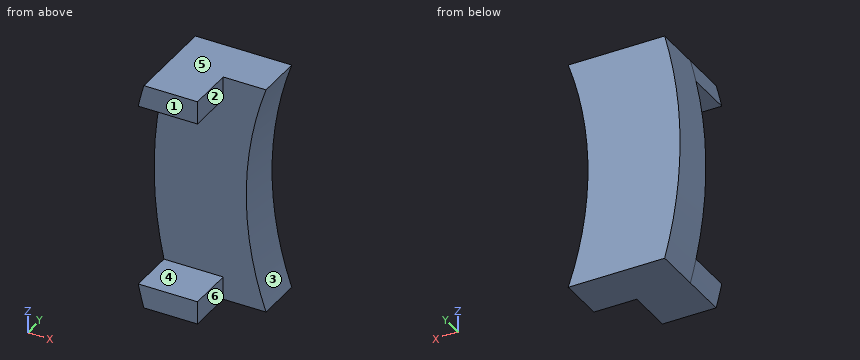
```python
from build123d import *

# Parameters (mm, degrees)
BOSS_EXTRUDE1_DEPTH = 2
BOSS_EXTRUDE2_DEPTH = 2


with BuildPart() as part:
    # Sketch1 → Boss-Extrude1 (new body)
    with BuildSketch(Plane(origin=(0, 0, 0), x_dir=(1, 0, 0), z_dir=(0, 1, 0))):
        with BuildLine():
            Line((-18.33030278, 5), (-14.142135624, 5))
            ThreePointArc((-14.142135624, 5), (-15, 0), (-14.142135624, -5))
            Line((-14.142135624, -5), (-18.33030278, -5))
            ThreePointArc((-18.33030278, -5), (-19, 0), (-18.33030278, 5))
        make_face()
    extrude(amount=BOSS_EXTRUDE1_DEPTH)

    # Sketch2 → Boss-Extrude2 (add)
    with BuildSketch(Plane.XZ):
        with BuildLine():
            Line((-16, -5), (-18.33030278, -5))
            ThreePointArc((-18.33030278, -5), (-18.459012203, -4.501651751), (-18.574175621, -4))
            Line((-18.574175621, -4), (-16, -4))
            Line((-16, -4), (-16, -5))
        make_face()
        with BuildLine():
            Line((-18.33030278, 5), (-16, 5))
            Line((-16, 5), (-16, 4))
            Line((-16, 4), (-18.574175621, 4))
            ThreePointArc((-18.574175621, 4), (-18.459012203, 4.501651751), (-18.33030278, 5))
        make_face()
    extrude(amount=BOSS_EXTRUDE2_DEPTH)


solid = part.part
```
CAD build for the part. Positions are in the model's coordinates, mm. Face numbers are marked on the shaded views. A direction names the side the tool comes from. Round coordinates to 2 decimals unless told otherwise and drop trailing zeros. Write each loop counter-clockwise with the first axis right and the second up, starting at its lowest first coordinate (ties: lowest second). Pieces come first, ordered by that corner, then holes. Notation, with made-up numbers: (-38, 82.5) -> (-22, 82.5) arc R16 cw to (-22, 95.5) -> close; hole circle Ø8 at (85, -18). An arc over 180 degrees is marked (long way). Answer in a Markdown table with one row per item. Add a question column.
Item 1: Mould opens along Z. For the marked faces 3, 4, 5 and 6 say: pulls with the +Z half, pulls with the -Z half, needs draft (parallel to the pull), parting line crosses it, or undercut.
Item 2: Saw through at B-B, the plane x = -17.4. Write the cut outline in (y, z).
Item 3: Drop flat-ended pins along their axis: pin 1 Ø1 at (y, z) = (0.5, -4) entering from +X; pin 2 Ø0.5 at (y, z) = (-1.5, -4.5) entering from +X; pin 3 Ø1 at (x, z) = (-16, -0.5) entering from -Y. Give the stop position or say it passes through.
Item 4: Drill centre lines: line 1 (Z direction, x = -17.2, y = -1.75); line 2 (Y direction, x = -18.3, z = 1); line 3 (X direction, y = 0.3, z = -0.75). Where is each one in solid material? Low to high. Write a range as from..to.
Item 5: Saw through at C-C, the plane x = -14.45. Write the cut outline in (y, z), then the cut area to 3 significant figures.
Item 6: Which spindle directions (+Z, -Z, +X, -X, +Y, -Y) get a long thin tool onto all of the face, cutting with end or side? Do the marked faces 1 and 2. Say none if no direction does.
Item 7: Saw through at A-A, the plane y = -1.05. Write the cut outline in (x, z), then the cut area to 3 significant figures.
Item 8: Saw through at D-D, the plane z = 0. Write the cut outline in (x, y), then the cut area to 3 significant figures.
Findings below:
| question | item | result |
|---|---|---|
| 1 | face 3 | undercut |
| 1 | face 4 | undercut |
| 1 | face 5 | pulls with the +Z half |
| 1 | face 6 | needs draft |
| 2 | outline | (-2, -5) -> (2, -5) -> (2, 5) -> (-2, 5) -> (-2, 4) -> (0, 4) -> (0, -4) -> (-2, -4) -> close |
| 3 | pin 1 | stops at x = -14.31 |
| 3 | pin 2 | stops at x = -16 |
| 3 | pin 3 | stops at y = 0 |
| 4 | line 1 | z = -5..-4, 4..5 |
| 4 | line 2 | y = 0..2 |
| 4 | line 3 | x = -18.99..-14.98 |
| 5 | outline | (0, -5) -> (2, -5) -> (2, -4.02) -> (0, -4.02) -> close; (0, 4.02) -> (2, 4.02) -> (2, 5) -> (0, 5) -> close |
| 5 | area | 3.90 mm^2 |
| 6 | face 1 | +Z, -Z, +X, -X, -Y |
| 6 | face 2 | +Z, -Z, +X, -Y |
| 7 | outline | (-18.57, -4) arc R19 ccw to (-18.33, -5) -> (-16, -5) -> (-16, -4) -> close; (-18.57, 4) -> (-16, 4) -> (-16, 5) -> (-18.33, 5) arc R19 ccw to start |
| 7 | area | 4.91 mm^2 |
| 8 | outline | (-19, 0) -> (-15, 0) -> (-15, 2) -> (-19, 2) -> close |
| 8 | area | 8.00 mm^2 |
